CAD build for the part. Positions are in the model's coordinates, mm. Face numbers are marked on the shaded views. A direction names the side the tool comes from. Round coordinates to 2 decimals unless told otherwise and drop trailing zeros. Order: outer loops, then holes, each group sorted by start corner. A loop starts at its lowest first (then second) coordinate and runs counter-clockwise, first axis right, second up. Notation, with made-up numbers: (-3, 44) -> (53, 44) arc R23 ccw to (53, 60) -> close; hole circle Ø6 at (39, 85). An arc over 180 degrees is marked (long way). Return JSON: item names as keys, results as strings. Group by question number.
Q1. Probe line 1 along Y through (x, z) = (0, -1.5); line 2 along X through (y, z) = (0, 9.75) (3 decimals); line 3 along X through (y, z) = (0, 18.5). List the from-to ranges inside material, lowest first.
Q2. Cut at C-C (z = 9). Write the cut outline in (x, y) (3 decimals).
Q3. Which spindle directions (+Z, -Z, +X, -X, +Y, -Y) get a long thin tool onto all of the face, cutting with end or side? Do the marked faces 3, 4 and 5. Say none if no direction does.
Q4. Flat gauge pins, fed straight in: pin 1 (2 mm diameter, centred on y = -9, z = 20, fed in from -X); pin 2 (6 mm diameter, centred on x = -6, z = 2.5, fed in from +Y); pin 3 (8 mm diameter, centred on x = -5, y = 4, fed in from -Z); pin 4 (2 mm diameter, centred on y = 1, z = 2.5, fed in from -X). Where does each tip first touch, or does it go through?
Q5. Mould opens along X. For the marked faces 1 and 2 say: +X half, -X half, draft (parallel to the pull), parting line (faces both ways), or undercut.
Q6. Cut at A-A (y = 0). Write the cut outline in (x, z) (1 decimal), then the cut area to 3 significant figures.
from build123d import *

# Parameters (mm, degrees)
F2_SIZE = 1.016


with BuildPart() as f1:
    # F0 (on Front) → F1 (revolve)
    with BuildSketch(Plane.XZ):
        Polygon((11.1125, 25.053447), (11.1125, 23.840199), (11.1125, 16.855199), (9.525, 16.855199), (9.525, 3.266199), (11.1125, 3.266199), (11.1125, -3.718801), (11.6205, -3.718801), (11.6205, 1.812447), (13.081, 1.812447), (13.081, 25.053447), align=None)
    revolve(axis=Axis((0, 0, -1.874024), (0, 0, -1)))

    # F2
    f2_edges = [f1.edges().sort_by_distance(p)[0] for p in [
        (-11.1125, 0, 25.053447),
    ]]
    chamfer(f2_edges, length=F2_SIZE)


solid = f1.part
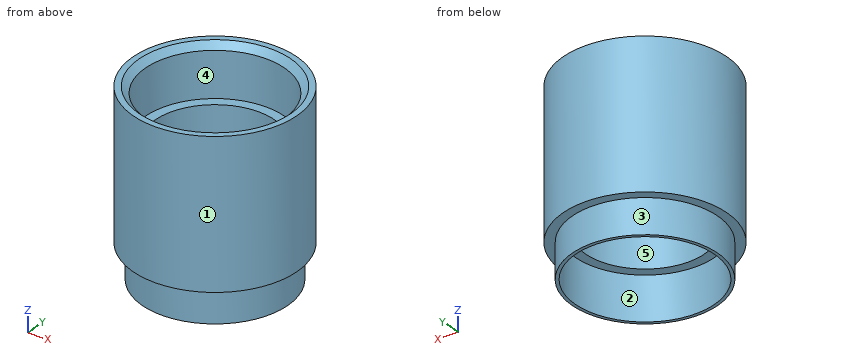
Solution:
{
 "1": {"line 1": "y = -11.62 to -11.11, 11.11 to 11.62", "line 2": "x = -13.081 to -9.525, 9.525 to 13.081", "line 3": "x = -13.08 to -11.11, 11.11 to 13.08"},
 "2": {"outline": "circle Ø26.162 at (0, 0); hole circle Ø19.05 at (0, 0)"},
 "3": {"face 3": "-Z", "face 4": "+Z", "face 5": "+Z, -Z"},
 "4": {"pin 1": "stops at x = -10.35", "pin 2": "stops at y = 12.73", "pin 3": "stops at z = 3.27", "pin 4": "stops at x = -13.08"},
 "5": {"face 1": "parting line", "face 2": "undercut"},
 "6": {"outline": "(-13.1, 1.8) -> (-11.6, 1.8) -> (-11.6, -3.7) -> (-11.1, -3.7) -> (-11.1, 3.3) -> (-9.5, 3.3) -> (-9.5, 16.9) -> (-11.1, 16.9) -> (-11.1, 24) -> (-12.1, 25.1) -> (-13.1, 25.1) -> close; (9.5, 3.3) -> (11.1, 3.3) -> (11.1, -3.7) -> (11.6, -3.7) -> (11.6, 1.8) -> (13.1, 1.8) -> (13.1, 25.1) -> (12.1, 25.1) -> (11.1, 24) -> (11.1, 16.9) -> (9.5, 16.9) -> close", "area": "139 mm²"}
}
